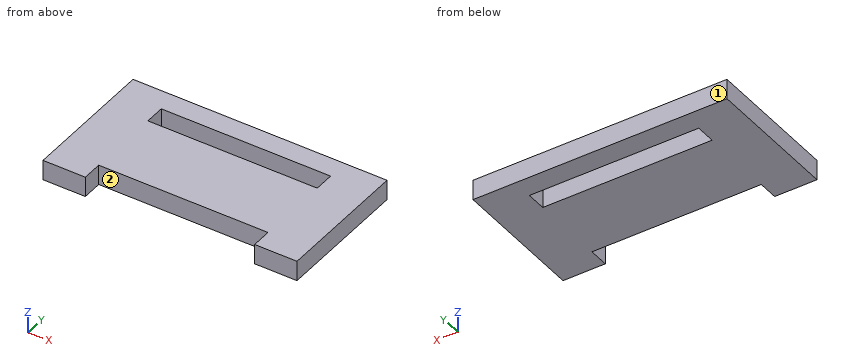
from build123d import *

# Parameters (mm, degrees)
BOSS_EXTRUDE1_DEPTH = 4.75
SKETCH2_W           = 60
SKETCH2_H           = 4.75
BOSS_EXTRUDE2_DEPTH = 5


with BuildPart() as part:
    # Sketch1 → Boss-Extrude1 (new body)
    with BuildSketch(Plane.XY):
        Polygon((0, 0), (10, 0), (10, 4.75), (50, 4.75), (50, 0), (60, 0), (60, 27), (50, 27), (50, 22.25), (10, 22.25), (10, 27), (0, 27), align=None)
    extrude(amount=BOSS_EXTRUDE1_DEPTH)

    # Sketch2 → Boss-Extrude2 (add)
    with BuildSketch(Plane(origin=(0, 27, 0), x_dir=(1, 0, 0), z_dir=(0, 1, 0))):
        with Locations((30, -2.375)):
            Rectangle(SKETCH2_W, SKETCH2_H)
    extrude(amount=BOSS_EXTRUDE2_DEPTH)


solid = part.part
Could you check a few things on this model? Use its own coordinates, in mm. Face numbers are marked on the shaded views. Coordinates: 2 decimals unless noted, no trailing zeros. Loops run counter-clockwise (first coordinate to the right, second up) from the corner with the lowest first, then second, coordinate; pieces in that order, holes last.
1. Imagine slicing it at C-C (z = 3.75). Please give me the cut outline in (x, y), and give its area (3 significant figures).
2. I need wall thicknesses on L1, parallel to X at y = 2, z = 4.5; L2, parallel to Y at x = 23, z = 0.4. Which ranges of each line are inside material? Lowest first, please.
3. We'd pull the mould along X, two halves only. Please class the marked faces 1 and 2: released by +X, released by -X, zero draft, split by the parting line, or undercut.
4. For P1, Ø5, axis at x = 30, y = 10.5, coming from the -Z side; P2, Ø1.4, axis at x = 29, z = 2.5, coming from the -Y side, each with a flat end and sliding along its axis, tell me the tip position at first contact or that it passes through.
5. Imagine slicing it at A-A (x = 28.5). Please give me the cut outline in (y, z).
6. Imagine slicing it at B-B (y = 26). Please give me the cut outline in (x, z), and give its area (3 significant figures).
Computed values:
1. outline: (0, 0) - (10, 0) - (10, 4.75) - (50, 4.75) - (50, 0) - (60, 0) - (60, 32) - (0, 32) - close; hole (10, 22.25) - (50, 22.25) - (50, 27) - (10, 27) - close
1. area: 1,540 mm2
2. L1: x = 0 to 10, 50 to 60
2. L2: y = 4.75 to 22.25, 27 to 32
3. face 1: zero draft
3. face 2: undercut
4. P1: stops at z = 0
4. P2: stops at y = 4.75
5. outline: (4.75, 0) - (22.25, 0) - (22.25, 4.75) - (4.75, 4.75) - close; (27, 0) - (32, 0) - (32, 4.75) - (27, 4.75) - close
6. outline: (0, 0) - (10, 0) - (10, 4.75) - (0, 4.75) - close; (50, 0) - (60, 0) - (60, 4.75) - (50, 4.75) - close
6. area: 95.0 mm2
